Answer from the drawing. Dimensions are ordinates in mm from the lowest x, y and z of the part. Give positions to 0.01 mm unless a question says otherwise; leave off trailing zeros. Write each loop counter-clockwise with the first axis right and the second up, starting at its lowest first coordinate (ties: lowest second). Pieces come first, ordered by that corner, then holes. Notation, with made-up numbers: (-0.75, 14) - (32.25, 14) arc R10 cw to (32.25, 20) - close; hole circle Ø9 at (31.5, 19.5). An arc over 180 degrees is marked (long way). Answer as a JSON object with one key per item and string values. Group by question number.
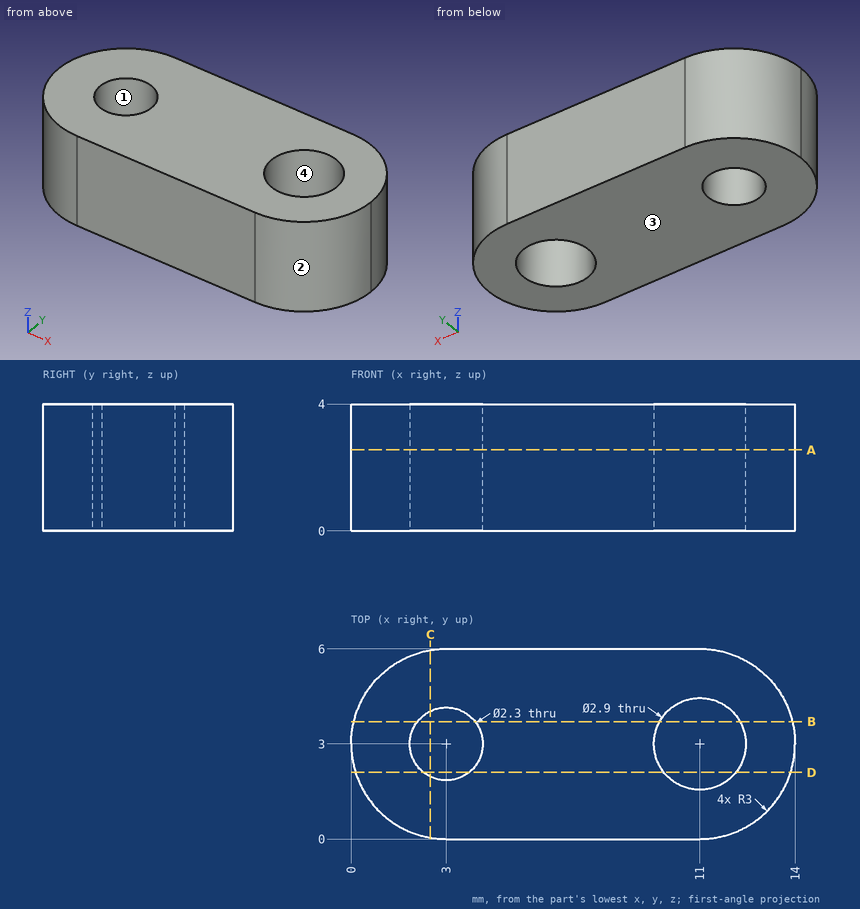
1) Find the intervals of material crossed by line 1 (X direction, y = 3, z = 1.65); line 2 (Y direction, x = 11, z = 0.95); line 3 (Y direction, x = 3, z = 1.8), in increasing order. Write a range as [from, to].
2) For a pull along X with two mould halves and no side action, classify the marked faces 1, 2, 3 and 4 as released by +X, released by -X, zero draft, split by the parting line, or undercut.
3) Find section C-C, the plane x = 2.5. Write down the section's boundary in (y, z).
4) Find section D-D, the plane y = 2.1. Write down the section's boundary in (x, z).
5) Find section A-A, the plane z = 2.55. Give the number of separate pieces and of enclosed holes in the cut face, and give its area (3 significant figures).
6) A flat-ended cylindrical pin translates along its axis: pin 1 Ø1.5 at (y, z) = (1, 1) entering from +X. Find the tip coordinate at first contact, or state that the pin passes through.
7) Find section B-B, the plane y = 3.7. Write down the section's boundary in (x, z).
Values follow:
{
 "1": {"line 1": "x = [0, 1.85], [4.15, 9.55], [12.45, 14]", "line 2": "y = [0, 1.55], [4.45, 6]", "line 3": "y = [0, 1.85], [4.15, 6]"},
 "2": {"face 1": "undercut", "face 2": "released by +X", "face 3": "zero draft", "face 4": "undercut"},
 "3": {"outline": "(0.04, 0) - (1.96, 0) - (1.96, 4) - (0.04, 4) - close; (4.04, 0) - (5.96, 0) - (5.96, 4) - (4.04, 4) - close"},
 "4": {"outline": "(0.14, 0) - (2.28, 0) - (2.28, 4) - (0.14, 4) - close; (3.72, 0) - (9.86, 0) - (9.86, 4) - (3.72, 4) - close; (12.14, 0) - (13.86, 0) - (13.86, 4) - (12.14, 4) - close"},
 "5": {"separate pieces": "1", "enclosed holes": "2", "area": "65.5 mm2"},
 "6": {"pin 1": "stops at x = 13.73"},
 "7": {"outline": "(0.08, 0) - (2.09, 0) - (2.09, 4) - (0.08, 4) - close; (3.91, 0) - (9.73, 0) - (9.73, 4) - (3.91, 4) - close; (12.27, 0) - (13.92, 0) - (13.92, 4) - (12.27, 4) - close"}
}
